```python
from build123d import *

# Parameters (mm, degrees)
CYLINDER_R        = 5.2
CYLINDER_DEPTH    = 5
CYLINDER002_R     = 2.25
CYLINDER002_DEPTH = 15
ARRAY_COUNT       = 4
CYLINDER005_R     = 25
CYLINDER005_DEPTH = 2
CYLINDER001_R     = 15
CYLINDER001_DEPTH = 8
CHAMFER_SIZE      = 2.5


with BuildPart() as eje:
    # Cylinder → Cylinder (new body)
    with BuildSketch(Plane.XY):
        Circle(CYLINDER_R)
    extrude(amount=CYLINDER_DEPTH)


with BuildPart() as fusion:
    # Cylinder002 → Cylinder002 (new body)
    with BuildSketch(Plane(origin=(8, 0, 0), x_dir=(1, 0, 0), z_dir=(0, 0, 1))):
        Circle(CYLINDER002_R)
    extrude(amount=CYLINDER002_DEPTH)

    # Array: Fusion ×4 about axis
    array_axis = Axis((0, 0, 0), (0, 0, 1))


with BuildPart() as fusion_1:
    add(fusion.part)
    for i in range(1, ARRAY_COUNT):
        add(fusion.part.rotate(array_axis, i * 360 / ARRAY_COUNT))

    # Fusion: union eje
    add(eje.part)


with BuildPart() as cilindro003:
    # Cylinder005 → Cylinder005 (new body)
    with BuildSketch(Plane.XY):
        Circle(CYLINDER005_R)
    extrude(amount=CYLINDER005_DEPTH)


with BuildPart() as cono:
    # Cone → Cone (revolve)
    with BuildSketch(Plane(origin=(0, 0, 2), x_dir=(1, 0, 0), z_dir=(0, -1, 0))):
        Polygon((0, 0), (25, 0), (15, 6), (0, 6), align=None)
    revolve(axis=Axis((0, 0, 2), (0, 0, 1)))


with BuildPart() as chamfer_body:
    # Cylinder001 → Cylinder001 (new body)
    with BuildSketch(Plane.XY):
        Circle(CYLINDER001_R)
    extrude(amount=CYLINDER001_DEPTH)

    # Fusion001: union Cilindro003, Cono
    add(cilindro003.part)
    add(cono.part)

    # Cut: cut Fusion
    add(fusion_1.part, mode=Mode.SUBTRACT)

    # Chamfer
    chamfer_edges = [chamfer_body.edges().sort_by_distance(p)[0] for p in [
        (5.75, 0, 8),
        (0, -5.75, 8),
        (-5.75, 0, 8),
        (0, 5.75, 8),
    ]]
    chamfer(chamfer_edges, length=CHAMFER_SIZE)


solid = chamfer_body.part
```
Verification items for the finished model (mm, model axes). A direction names the side the tool comes from. Coordinates: 2 decimals unless noted, no trailing zeros. Order: outer loops, then holes, each group sorted by start corner. A loop starts at its lowest first (then second) coordinate and runs counter-clockwise, first axis right, second up. Notation, with made-up numbers: (83.25, 19.25) -> (100.25, 19.25) arc R6 cw to (100.25, 25.25) -> close; hole circle Ø5 at (15, 20.25). An arc over 180 degrees is marked (long way). Put each result on its own line as item: value. Start each with the question number.
1) Cross-section at C-C (z = 7.25). Enter the section's corners in (x, y).
2) Material ranges on L1, parallel to Y at x = 1.5, z = 3.75; L2, parallel to X at y = -1.5, z = 3; L3, parallel to X at y = -8, z = 5.75, recorded low to high.
3) Go/stop test with flat-tipped pins: pin 1 (10 mm diameter, centred on x = -19.5, y = 14, fed in from +Z); pin 2 (7 mm diameter, centred on x = 8, y = 0, fed in from +Z); pin 3 (1.5 mm diameter, centred on x = 6, z = 4, fed in from -Y). Record where each tip stops, or that it passes through.
4) Cross-section at D-D (z = 3.75). Enter the section's corners in (x, y).
5) Release check for a two-part mould opening along Y. For faces 3 (the cylindrical face through (-0.099, 5.752, 2.712)), 4 (the flat face through (0, 0, 8)), 5 (the cylindrical face through (23.846, 7.509, 0.986)) record: pulls with the +Y half, pulls with the -Y half, needs draft (parallel to the pull), parting line crosses it, or undercut.
6) Tool access check on faces 1 (the cylindrical face through (-0.677, 5.156, 2.465)), 2 (the conical face through (10.26, -0.71, 5.62)). Record the directions out of +Z, -Z, +X, -X, +Y, -Y that give a thin tool (end or side, any length) a straight path to the whole face; none if there is none.
7) Cross-section at A-A (x = 0). Enter the section's corners in (y, z).
Geometry check:
1. outline: circle Ø32.5 at (0, 0); hole circle Ø8 at (-8, 0); hole circle Ø8 at (0, -8); hole circle Ø8 at (0, 8); hole circle Ø8 at (8, 0)
2. L1: y = -22.03 to -9.68, -6.32 to -4.98, 4.98 to 6.32, 9.68 to 22.03
2. L2: x = -23.29 to -9.68, -6.32 to -4.98, 4.98 to 6.32, 9.68 to 23.29
2. L3: x = -16.96 to -2.5, 2.5 to 16.96
3. pin 1: stops at z = 5.6
3. pin 2: stops at z = 6.75
3. pin 3: stops at y = -22.13
4. outline: circle Ø44.17 at (0, 0); hole circle Ø4.5 at (-8, 0); hole circle Ø10.4 at (0, 0); hole circle Ø4.5 at (0, -8); hole circle Ø4.5 at (0, 8); hole circle Ø4.5 at (8, 0)
5. face 3: undercut
5. face 4: needs draft
5. face 5: parting line crosses it
6. face 1: -Z
6. face 2: +Z
7. outline: (-25, 0) -> (-10.25, 0) -> (-10.25, 5.5) -> (-12.75, 8) -> (-15, 8) -> (-25, 2) -> close; (-5.75, 0) -> (-5.2, 0) -> (-5.2, 5) -> (5.2, 5) -> (5.2, 0) -> (5.75, 0) -> (5.75, 5.5) -> (3.25, 8) -> (-3.25, 8) -> (-5.75, 5.5) -> close; (10.25, 0) -> (25, 0) -> (25, 2) -> (15, 8) -> (12.75, 8) -> (10.25, 5.5) -> close
